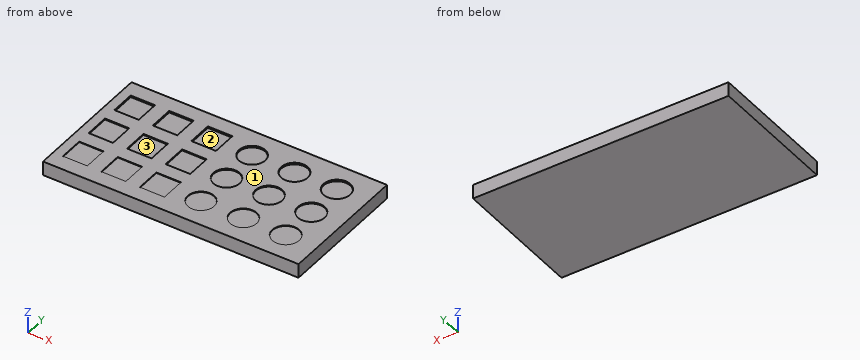
```python
from build123d import *

# Parameters (mm, degrees)
F3_W      = 452.06105
F3_H      = 233.740471
F4_DEPTH  = 25
F0_W      = 43
F0_H      = 43
F0_W_2    = 43.25
F0_H_2    = 43.25
F0_W_3    = 43.5
F0_H_3    = 43.5
F5_DEPTH  = 1
F1_W      = 43
F1_H      = 43
F1_W_2    = 43.25
F1_H_2    = 43.25
F1_W_3    = 43.5
F1_H_3    = 43.5
F6_DEPTH  = 2
F2_W      = 43
F2_H      = 43
F2_W_2    = 43.25
F2_H_2    = 43.25
F2_W_3    = 43.5
F2_H_3    = 43.5
F7_DEPTH  = 3
F8_R      = 23.25
F8_R_2    = 23.5
F8_R_3    = 23.75
F11_DEPTH = 1
F9_R      = 23.25
F9_R_2    = 23.5
F9_R_3    = 23.75
F12_DEPTH = 2
F10_R     = 23.25
F10_R_2   = 23.5
F10_R_3   = 23.75
F13_DEPTH = 3


with BuildPart() as f4:
    # F3 (on Top) → F4 (new body)
    with BuildSketch(Plane.XY):
        with Locations((187.43575, 68.15933)):
            Rectangle(F3_W, F3_H)
    extrude(amount=-F4_DEPTH)

    # F0 (on Top) → F5 (cut)
    with BuildSketch(Plane.XY):
        Rectangle(F0_W, F0_H)
        with Locations((68.125, 0)):
            Rectangle(F0_W_2, F0_H_2)
        with Locations((136.5, 0)):
            Rectangle(F0_W_3, F0_H_3)
    extrude(amount=-F5_DEPTH, mode=Mode.SUBTRACT)

    # F1 (on Top) → F6 (cut)
    with BuildSketch(Plane.XY):
        with Locations((0, 68)):
            Rectangle(F1_W, F1_H)
        with Locations((68.125, 68)):
            Rectangle(F1_W_2, F1_H_2)
        with Locations((136.5, 68)):
            Rectangle(F1_W_3, F1_H_3)
    extrude(amount=-F6_DEPTH, mode=Mode.SUBTRACT)

    # F2 (on Top) → F7 (cut)
    with BuildSketch(Plane.XY):
        with Locations((0, 136)):
            Rectangle(F2_W, F2_H)
        with Locations((68.125, 136)):
            Rectangle(F2_W_2, F2_H_2)
        with Locations((136.5, 136)):
            Rectangle(F2_W_3, F2_H_3)
    extrude(amount=-F7_DEPTH, mode=Mode.SUBTRACT)

    # F8 (on face) → F11 (cut)
    with BuildSketch(Plane.XY):
        with Locations((208.25, 0)):
            Circle(F8_R)
        with Locations((283.25, 0)):
            Circle(F8_R_2)
        with Locations((358.25, 0)):
            Circle(F8_R_3)
    extrude(amount=-F11_DEPTH, mode=Mode.SUBTRACT)

    # F9 (on face) → F12 (cut)
    with BuildSketch(Plane.XY):
        with Locations((208.25, 67.5)):
            Circle(F9_R)
        with Locations((283.25, 67.5)):
            Circle(F9_R_2)
        with Locations((358.25, 67.5)):
            Circle(F9_R_3)
    extrude(amount=-F12_DEPTH, mode=Mode.SUBTRACT)

    # F10 (on face) → F13 (cut)
    with BuildSketch(Plane.XY):
        with Locations((208.25, 135)):
            Circle(F10_R)
        with Locations((283.25, 135)):
            Circle(F10_R_2)
        with Locations((358.25, 135)):
            Circle(F10_R_3)
    extrude(amount=-F13_DEPTH, mode=Mode.SUBTRACT)


solid = f4.part
```
The listing builds one solid part. Answer for the finished solid, in the listing's coordinates (mm). Face numbers are marked on the shaded views. Give positions to 0.01 mm unless a question says otherwise; leave off trailing zeros. Order: outer loops, then holes, each group sorted by start corner. A loop starts at its lowest first (then second) coordinate and runs counter-clockwise, first axis right, second up. Notation, with made-up numbers: M 33.25,88 L 54.25,88 A13 ccw 54.25,95 Z; hole C -37,18.5 d3. An arc over 180 degrees is marked long. Put each result on its own line as item: value. Start each with the question number.
Item 1: Find the intervals of material crossed by line 1 along Y through (x, z) = (358.25, -0.5); line 2 along Y through (x, z) = (208.25, -0.5); line 3 along Y through (x, z) = (358.25, -1.8), in increasing order.
Item 2: The part is cut by section B-B, the plane x = 208.25. Determine the outline of the cut face in (y, z).
Item 3: The part is cut by section A-A, the plane y = 0. Determine the outline of the cut face in (x, z), and give its area (3 significant figures).
Item 4: The part is cut by section D-D, the plane y = 67.5. Determine the outline of the cut face in (x, z).
Item 5: For a pull along Y with two mould halves and no side action, classify the marked faces 1, 2 and 3 as +Y half, -Y half, draft (parallel to the pull), parting line (faces both ways), or undercut.
Item 6: A flat-ended cylindrical pin translates along its axis: P1, Ø14, axis at x = 368, y = 71, coming from the +Z side. Find the tip coordinate at first contact, or state that the pin passes through.
Item 7: The part is cut by section C-C, the plane x = 73. Determine the outline of the cut face in (y, z) (3 decimals).
Answer key:
1. line 1: y = -48.71 to -23.75, 23.75 to 43.75, 91.25 to 111.25, 158.75 to 185.03
1. line 2: y = -48.71 to -23.25, 23.25 to 44.25, 90.75 to 111.75, 158.25 to 185.03
1. line 3: y = -48.71 to 43.75, 91.25 to 111.25, 158.75 to 185.03
2. outline: M -48.71,-25 L 185.03,-25 L 185.03,0 L 158.25,0 L 158.25,-3 L 111.75,-3 L 111.75,0 L 90.75,0 L 90.75,-2 L 44.25,-2 L 44.25,0 L 23.25,0 L 23.25,-1 L -23.25,-1 L -23.25,0 L -48.71,0 Z
3. outline: M -38.59,-25 L 413.47,-25 L 413.47,0 L 382,0 L 382,-1 L 334.5,-1 L 334.5,0 L 306.75,0 L 306.75,-1 L 259.75,-1 L 259.75,0 L 231.5,0 L 231.5,-1 L 185,-1 L 185,0 L 158.25,0 L 158.25,-1 L 114.75,-1 L 114.75,0 L 89.75,0 L 89.75,-1 L 46.5,-1 L 46.5,0 L 21.5,0 L 21.5,-1 L -21.5,-1 L -21.5,0 L -38.59,0 Z
3. area: 11,000 mm²
4. outline: M -38.59,-25 L 413.47,-25 L 413.47,0 L 382,0 L 382,-2 L 334.5,-2 L 334.5,0 L 306.75,0 L 306.75,-2 L 259.75,-2 L 259.75,0 L 231.5,0 L 231.5,-2 L 185,-2 L 185,0 L 158.25,0 L 158.25,-2 L 114.75,-2 L 114.75,0 L 89.75,0 L 89.75,-2 L 46.5,-2 L 46.5,0 L 21.5,0 L 21.5,-2 L -21.5,-2 L -21.5,0 L -38.59,0 Z
5. face 1: draft
5. face 2: undercut
5. face 3: undercut
6. P1: stops at z = -2
7. outline: M -48.711,-25 L 185.03,-25 L 185.03,0 L 157.625,0 L 157.625,-3 L 114.375,-3 L 114.375,0 L 89.625,0 L 89.625,-2 L 46.375,-2 L 46.375,0 L 21.625,0 L 21.625,-1 L -21.625,-1 L -21.625,0 L -48.711,0 Z
